Part print with two shaded views. Sizes in mm from the minimum x, y, z corner. A direction names the side the tool comes from. Coordinates: 2 decimals unless noted, no trailing zeros. Write each loop counter-clockwise with the first axis right and the second up, starting at its lowest first coordinate (ties: lowest second). Pieces come first, ordered by that corner, then holes.
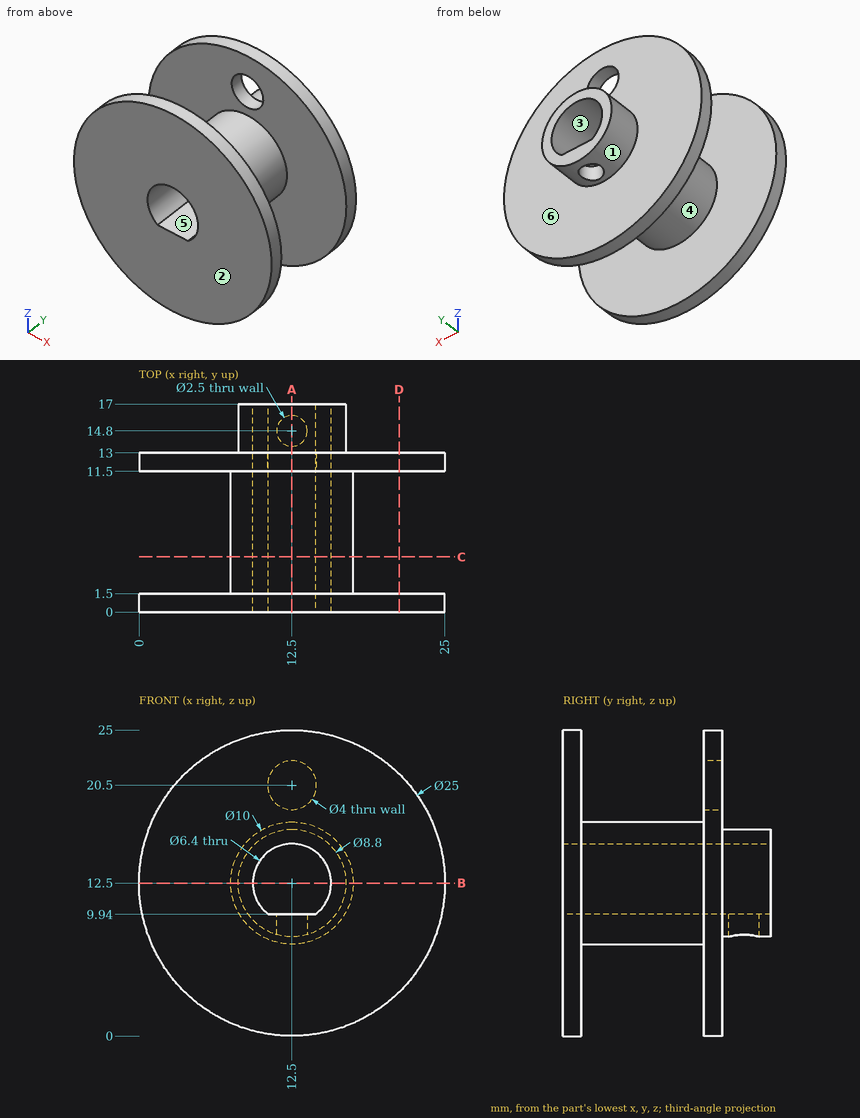
(1) Slice it at B-B, the plane z = 12.5. List the corners of the cut face in (x, y).
(2) Slice it at A-A, the plane x = 12.5. List the corners of the cut face in (y, z).
(3) Two-plate mould, pull along Z, no slides. Class the marked faces 1, 2 and 3: pulls with the +Z half, pulls with the -Z half, needs draft (parallel to the pull), parting line crosses it, or undercut.
(4) Flat gauge pins, fed straight in: P1, Ø3, axis at x = 12.5, y = 14.8, coming from the -Z side; P2, Ø2, axis at x = 19, y = 5.5, coming from the +Z side; P3, Ø5, axis at x = 16.5, y = 5, coming from the -Z side; P4, Ø10, axis at x = 8.5, z = 3, coming from the +Y side. Where does each tip first touch, or does it go through?
(5) Slice it at D-D, the plane x = 21.25. List the corners of the cut face in (y, z), and give its area (3 significant figures).
(6) Probe L1, parallel to Y at x = 23.75, z = 12.5; L2, parallel to Y at x = 12.5, z = 8.75; L3, parallel to X at y = 6, z = 12.5. List the from-to ranges inside material, lowest first.
(7) 3-axis set-ups, long thin cutter, end or side, ignore diameter. For the marked faces 4, 5 and 6: which of +Z, -Z, +X, -X, +Y, -Y reach the whole face in a straight line?
(8) Slice it at C-C, the plane y = 4.5. List the corners of the cut face in (x, z).
Results:
1. outline: (0, 0) - (9.3, 0) - (9.3, 17) - (8.1, 17) - (8.1, 13) - (0, 13) - (0, 11.5) - (7.5, 11.5) - (7.5, 1.5) - (0, 1.5) - close; (15.7, 0) - (25, 0) - (25, 1.5) - (17.5, 1.5) - (17.5, 11.5) - (25, 11.5) - (25, 13) - (16.9, 13) - (16.9, 17) - (15.7, 17) - close
2. outline: (0, 0) - (1.5, 0) - (1.5, 7.5) - (11.5, 7.5) - (11.5, 0) - (13, 0) - (13, 8.1) - (13.55, 8.1) - (13.55, 9.94) - (0, 9.94) - close; (0, 15.7) - (17, 15.7) - (17, 16.9) - (13, 16.9) - (13, 18.5) - (11.5, 18.5) - (11.5, 17.5) - (1.5, 17.5) - (1.5, 25) - (0, 25) - close; (11.5, 22.5) - (13, 22.5) - (13, 25) - (11.5, 25) - close; (16.05, 8.1) - (17, 8.1) - (17, 9.94) - (16.05, 9.94) - close
3. face 1: parting line crosses it
3. face 2: needs draft
3. face 3: undercut
4. P1: stops at z = 8.1
4. P2: passes through
4. P3: stops at z = 7.73
4. P4: stops at y = 13
5. outline: (0, 3.57) - (1.5, 3.57) - (1.5, 21.43) - (0, 21.43) - close; (11.5, 3.57) - (13, 3.57) - (13, 21.43) - (11.5, 21.43) - close
5. area: 53.6 mm2
6. L1: y = 0 to 1.5, 11.5 to 13
6. L2: y = 0 to 13.55, 16.05 to 17
6. L3: x = 7.5 to 9.3, 15.7 to 17.5
7. face 4: none
7. face 5: +Y, -Y
7. face 6: +Y
8. outline: circle Ø10 at (12.5, 12.5); hole (10.58, 9.94) - (14.42, 9.94) arc R3.2 ccw (long way) to start
